CAD build for the part. Positions are in the model's coordinates, mm. A direction names the side the tool comes from. Coordinates: 2 decimals unless noted, no trailing zeros. Write each loop counter-clockwise with the first axis right and the second up, starting at its lowest first coordinate (ties: lowest second). Pieces come first, ordered by that corner, then holes. Notation, with made-up numbers: M 22.5,-34 L 61.5,-34 A13 cw 61.5,-13 Z; hole C -2.75,-19 d6. An arc over 180 degrees is marked long. Answer as CSV lines item,"result". Start each with the question number.
```python
from build123d import *

# Parameters (mm, degrees)
RESSALTO_EXTRUS_O1_DEPTH = 1.5
FILETE1_R                = 3


with BuildPart() as part:
    # Esboço1 → Ressalto-extrusão1 (new, symmetric)
    with BuildSketch(Plane.XY):
        Polygon((-6.5, -8), (-6.5, 8), (6.5, 8), (12.323523748, -8), (3.5, -8), (3.5, -11), (-3.5, -11), (-3.5, -8), align=None)
    extrude(amount=RESSALTO_EXTRUS_O1_DEPTH, both=True)

    # Filete1
    filete1_edges = [part.edges().sort_by_distance(p)[0] for p in [
        (-6.5, 8, 0),
        (6.5, 8, 0),
    ]]
    fillet(filete1_edges, radius=FILETE1_R)


solid = part.part
```
1) Band-saw the part on C-C, the plane x = 4. List the corners of the cut face in (y, z).
2) Probe L1, parallel to X at y = -8.75, z = 1.1; L2, parallel to X at y = -0.75, z = -1; L3, parallel to Y at x = 6, z = 1.35. List the from-to ranges inside material, lowest first. Write a range as [from, to].
3) Pin check, flat tips, straight feed: P1, Ø2, axis at x = 7.5, y = -8.5, coming from the -Z side; P2, Ø0.9, axis at x = 9.5, z = 0.5, coming from the -Y side; P3, Ø1.5, axis at y = -9, z = 0.5, coming from the -X side. Stop position of each tip, or through.
4) Band-saw the part on B-B, the plane y = -8.5. List the corners of the cut face in (x, z), plus the area to 3 significant figures.
5) Tool access for faces 1 (the flat face through (-5, -8, 0)), 2 (the flat face through (8, -8, 0)), 3 (the cylindrical face through (6.141, 7.443, -0.021)): list every direction of +Z, -Z, +X, -X, +Y, -Y with a clear straight run to the whole face (end or side of a thin tool).
6) Band-saw the part on A-A, the plane z = 0.25. List the corners of the cut face in (x, y).
Result sheet:
1,outline,"M -8,-1.5 L 8,-1.5 L 8,1.5 L -8,1.5 Z"
2,L1,"x = [-3.5, 3.5]"
2,L2,"x = [-6.5, 9.68]"
2,L3,"y = [-8, 7.54]"
3,P1,"stops at z = -1.5"
3,P2,"stops at y = -8"
3,P3,"stops at x = -3.5"
4,outline,"M -3.5,-1.5 L 3.5,-1.5 L 3.5,1.5 L -3.5,1.5 Z"
4,area,"21.0 mm²"
5,face 1,"+Z, -Z, -X, -Y"
5,face 2,"+Z, -Z, +X, -Y"
5,face 3,"+Z, -Z, +X, +Y"
6,outline,"M -6.5,-8 L -3.5,-8 L -3.5,-11 L 3.5,-11 L 3.5,-8 L 12.32,-8 L 7.22,6.03 A3 ccw 4.4,8 L -3.5,8 A3 ccw -6.5,5 Z"
